The figure shows three views and two pictorial views of one solid part (mm, origin at its lowest corner). Answer the questions. Coordinates: 2 decimals unless noted, no trailing zeros. Write each loop counter-clockwise with the first axis right and the second up, starting at its lowest first coordinate (ties: lowest second). Pieces come first, ordered by that corner, then holes. Notation, with made-up numbers: M -6,7.5 L 52,7.5 A21 cw 52,33.5 Z; hole C 5,72.5 d6. An arc over 180 degrees is marked long. Use CSV: the item, a comma, the result in double quotes.
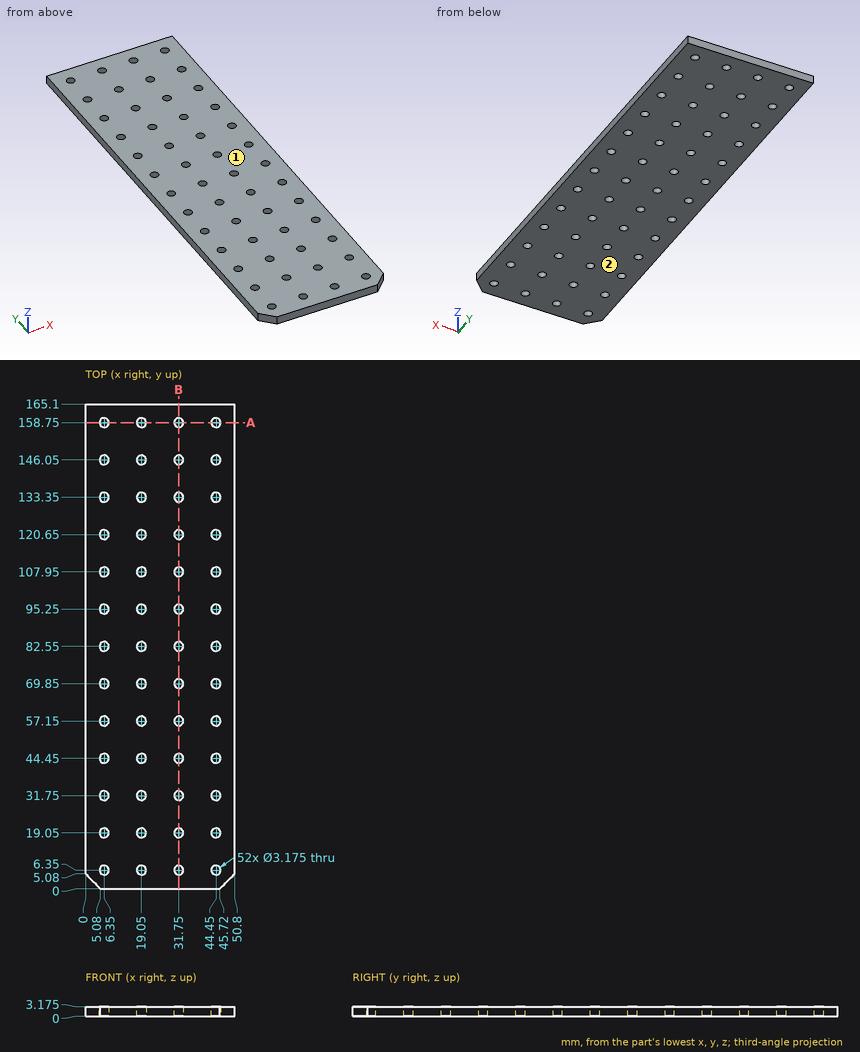
Item 1: The part is cut by section A-A (y = 158.75). Write down the section's boundary in (x, z) (1 decimal), then the cut area to 3 significant figures.
Answer:
outline,"M 0,0 L 4.8,0 L 4.8,3.2 L 0,3.2 Z; M 7.9,0 L 17.5,0 L 17.5,3.2 L 7.9,3.2 Z; M 20.6,0 L 30.2,0 L 30.2,3.2 L 20.6,3.2 Z; M 33.3,0 L 42.9,0 L 42.9,3.2 L 33.3,3.2 Z; M 46,0 L 50.8,0 L 50.8,3.2 L 46,3.2 Z"
area,"121 mm2"
Item 2: For a pull along Z with two mould halves and no side action, classify the marked faces 1 and 2 as released by +Z, released by -Z, zero draft, split by the parting line, or undercut.
Answer:
face 1,"released by +Z"
face 2,"released by -Z"
Item 3: Consider probe 1 along X at (y, z) = (44.45, 0.8); probe 2 along Y at (x, z) = (2.5, 2.05); probe 3 along Y at (x, z) = (46.5, 2.15). Determine where each line is inside the solid, lowest interval first.
Answer:
probe 1,"x = 0 to 4.76, 7.94 to 17.46, 20.64 to 30.16, 33.34 to 42.86, 46.04 to 50.8"
probe 2,"y = 2.58 to 165.1"
probe 3,"y = 0.78 to 165.1"
Item 4: Given pin 1 (1.9 mm diameter, centred on x = 44.45, y = 6.35, fed in from -Z), flat-ended and moving along its own axis, determine where the tip first touches the part or whether it passes through.
Answer:
pin 1,"passes through"
Item 5: The part is cut by section B-B (x = 31.75). Count the separate pieces of the cut face and the enclosed holes in it, then the cut area to 3 significant figures.
Answer:
separate pieces,"14"
enclosed holes,"0"
area,"393 mm2"
